The model under review builds one solid part; all positions refer to its coordinate system, in mm. A direction names the side the tool comes from. Coordinates: 2 decimals unless noted, no trailing zeros. Write each loop counter-clockwise with the first axis right and the second up, starting at its lowest first coordinate (ties: lowest second). Pieces come first, ordered by that corner, then holes.
```python
from build123d import *

# Parameters (mm, degrees)
F0_W     = 273
F0_H     = 229
F0_W_2   = 50
F0_H_2   = 60
F1_DEPTH = 2
F2_W     = 273
F2_H     = 229
F2_W_2   = 269
F2_H_2   = 225
F3_DEPTH = 25
F4_W     = 54
F4_H     = 64
F4_W_2   = 50
F4_H_2   = 60
F5_DEPTH = 30


with BuildPart() as f1:
    # F0 (on Top) → F1 (new body)
    with BuildSketch(Plane.XY):
        with Locations((133.5, 111.5)):
            Rectangle(F0_W, F0_H)
        with Locations((33.375, 37.167333)):
            Rectangle(F0_W_2, F0_H_2, mode=Mode.SUBTRACT)
        with Locations((100.125, 37.167333)):
            Rectangle(F0_W_2, F0_H_2, mode=Mode.SUBTRACT)
        with Locations((166.875, 37.167333)):
            Rectangle(F0_W_2, F0_H_2, mode=Mode.SUBTRACT)
        with Locations((233.625, 37.167333)):
            Rectangle(F0_W_2, F0_H_2, mode=Mode.SUBTRACT)
        with Locations((33.375, 111.500333)):
            Rectangle(F0_W_2, F0_H_2, mode=Mode.SUBTRACT)
        with Locations((100.125, 111.500333)):
            Rectangle(F0_W_2, F0_H_2, mode=Mode.SUBTRACT)
        with Locations((33.375, 185.833333)):
            Rectangle(F0_W_2, F0_H_2, mode=Mode.SUBTRACT)
        with Locations((100.125, 185.833333)):
            Rectangle(F0_W_2, F0_H_2, mode=Mode.SUBTRACT)
        with Locations((166.875, 111.500333)):
            Rectangle(F0_W_2, F0_H_2, mode=Mode.SUBTRACT)
        with Locations((233.625, 111.500333)):
            Rectangle(F0_W_2, F0_H_2, mode=Mode.SUBTRACT)
        with Locations((166.875, 185.833333)):
            Rectangle(F0_W_2, F0_H_2, mode=Mode.SUBTRACT)
        with Locations((233.625, 185.833333)):
            Rectangle(F0_W_2, F0_H_2, mode=Mode.SUBTRACT)
    extrude(amount=F1_DEPTH)

    # F2 (on face) → F3 (join)
    with BuildSketch(Plane.XY.offset(2)):
        with Locations((133.5, 111.5)):
            Rectangle(F2_W, F2_H)
        with Locations((133.5, 111.5)):
            Rectangle(F2_W_2, F2_H_2, mode=Mode.SUBTRACT)
    extrude(amount=F3_DEPTH)

    # F4 (on face) → F5 (join)
    with BuildSketch(Plane.XY.offset(2)):
        with Locations((33.375, 185.833333)):
            Rectangle(F4_W, F4_H)
        with Locations((33.375, 185.833333)):
            Rectangle(F4_W_2, F4_H_2, mode=Mode.SUBTRACT)
        with Locations((33.375, 111.500333)):
            Rectangle(F4_W, F4_H)
        with Locations((33.375, 111.500333)):
            Rectangle(F4_W_2, F4_H_2, mode=Mode.SUBTRACT)
        with Locations((33.375, 37.167333)):
            Rectangle(F4_W, F4_H)
        with Locations((33.375, 37.167333)):
            Rectangle(F4_W_2, F4_H_2, mode=Mode.SUBTRACT)
        with Locations((100.125, 185.833333)):
            Rectangle(F4_W, F4_H)
        with Locations((100.125, 185.833333)):
            Rectangle(F4_W_2, F4_H_2, mode=Mode.SUBTRACT)
        with Locations((100.125, 111.500333)):
            Rectangle(F4_W, F4_H)
        with Locations((100.125, 111.500333)):
            Rectangle(F4_W_2, F4_H_2, mode=Mode.SUBTRACT)
        with Locations((100.125, 37.167333)):
            Rectangle(F4_W, F4_H)
        with Locations((100.125, 37.167333)):
            Rectangle(F4_W_2, F4_H_2, mode=Mode.SUBTRACT)
        with Locations((166.875, 185.833333)):
            Rectangle(F4_W, F4_H)
        with Locations((166.875, 185.833333)):
            Rectangle(F4_W_2, F4_H_2, mode=Mode.SUBTRACT)
        with Locations((166.875, 111.500333)):
            Rectangle(F4_W, F4_H)
        with Locations((166.875, 111.500333)):
            Rectangle(F4_W_2, F4_H_2, mode=Mode.SUBTRACT)
        with Locations((166.875, 37.167333)):
            Rectangle(F4_W, F4_H)
        with Locations((166.875, 37.167333)):
            Rectangle(F4_W_2, F4_H_2, mode=Mode.SUBTRACT)
        with Locations((233.625, 185.833333)):
            Rectangle(F4_W, F4_H)
        with Locations((233.625, 185.833333)):
            Rectangle(F4_W_2, F4_H_2, mode=Mode.SUBTRACT)
        with Locations((233.625, 111.500333)):
            Rectangle(F4_W, F4_H)
        with Locations((233.625, 111.500333)):
            Rectangle(F4_W_2, F4_H_2, mode=Mode.SUBTRACT)
        with Locations((233.625, 37.167333)):
            Rectangle(F4_W, F4_H)
        with Locations((233.625, 37.167333)):
            Rectangle(F4_W_2, F4_H_2, mode=Mode.SUBTRACT)
    extrude(amount=F5_DEPTH)


solid = f1.part
```
Item 1: Machinability: for faces 3 (the face through (100, 217.833, 17)), 4 (the face through (8.375, 37, 16)), which of the approach directions +Z, -Z, +X, -X, +Y, -Y give a long, thin tool a straight path to every point of the face, cutting with its end or side? Answer none if there is none.
Solved:
face 3: +Z
face 4: +Z, -Z
Item 2: Take a section at C-C, the plane x = 132.5. Write out the cut boundary in (y, z), plus the area to 3 significant figures.
Solved:
outline: (-3, 0) - (226, 0) - (226, 27) - (224, 27) - (224, 2) - (-1, 2) - (-1, 27) - (-3, 27) - close
area: 558 mm2
Item 3: Take a section at A-A, the plane x = 242.5. Count the separate pieces of the cut face and the enclosed holes in it, plus the area to 3 significant figures.
Solved:
separate pieces: 4
enclosed holes: 0
area: 558 mm2
Item 4: Mouldability with a two-part tool opening along X and no side actions: class faces 1 (the face through (58.375, 37, 16)), 2 (the face through (133, 121, 0)) as pulls with the +X half, pulls with the -X half, needs draft (parallel to the pull), parting line crosses it, or undercut.
Solved:
face 1: undercut
face 2: needs draft
Item 5: To check wall thickness, follow line 1 along X through (y, z) = (167, 1.5) (3 decimals); line 2 along Y through (x, z) = (78, 31.5); line 3 along Y through (x, z) = (140.5, 17.5). State the ranges of each line that lie inside material, in increasing order.
Solved:
line 1: x = -3 to 8.375, 58.375 to 75.125, 125.125 to 141.875, 191.875 to 208.625, 258.625 to 270
line 2: y = 5.17 to 7.17, 67.17 to 69.17, 79.5 to 81.5, 141.5 to 143.5, 153.83 to 155.83, 215.83 to 217.83
line 3: y = -3 to -1, 5.17 to 69.17, 79.5 to 143.5, 153.83 to 217.83, 224 to 226
